Can you work these out from the drawing? Everything is in mm from the part's minimum corner. Give positions to 0.01 mm unless a question says otherwise; leave off trailing zeros. Loops run counter-clockwise (first coordinate to the right, second up) from the corner with the lowest first, then second, coordinate; pieces in that order, holes last. Notation, with made-up numbers: M 33.5,3 L 63.5,3 A10 cw 63.5,10 Z; hole C 36,-10 d4. An arc over 180 degrees is marked long. Use CSV: the item, a comma, the result in double quotes.
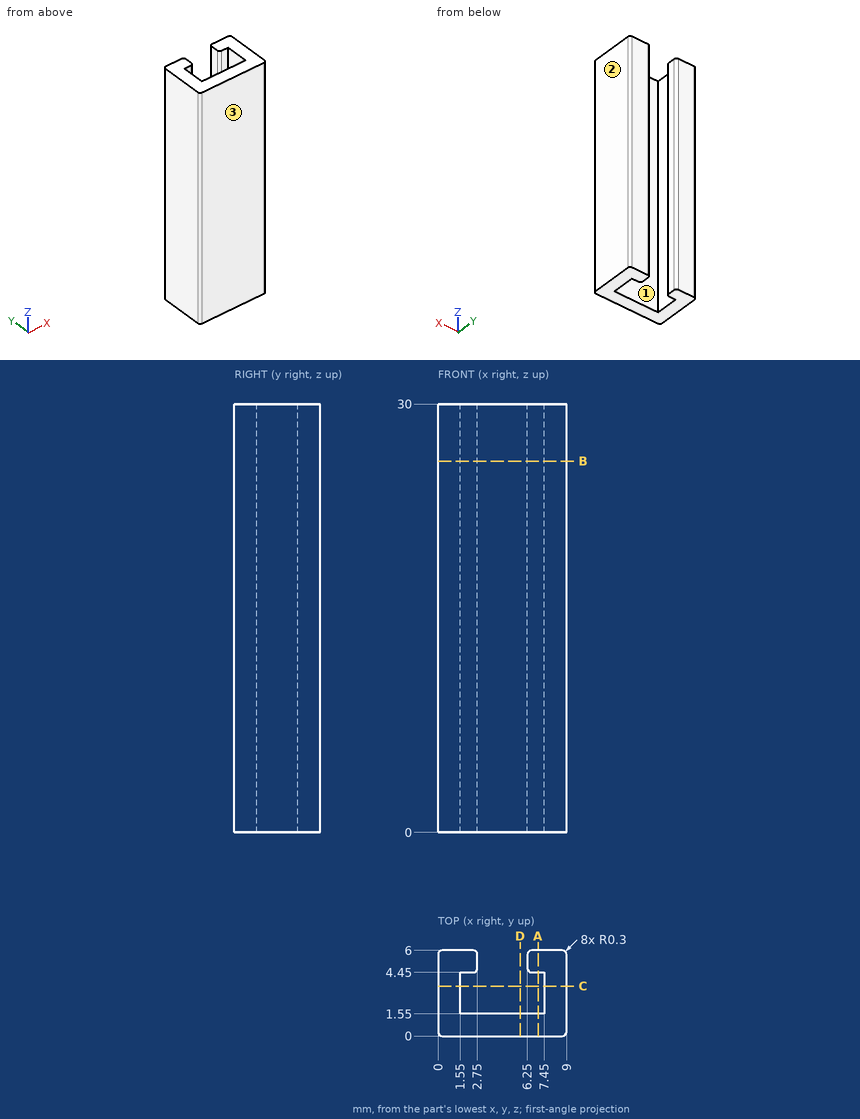
Q1. If we mould it in two halves opening along X, with no side actions, what happens to the marked faces 1, 2 and 3? For each: released by +X, released by -X, zero draft, split by the parting line, or undercut.
Model answer:
face 1,"undercut"
face 2,"released by +X"
face 3,"zero draft"
Q2. I want a section at A-A, the plane x = 7. Please give me the cut outline in (y, z).
Model answer:
outline,"M 0,0 L 1.55,0 L 1.55,30 L 0,30 Z; M 4.45,0 L 6,0 L 6,30 L 4.45,30 Z"
Q3. Please list where these lines run through material, in increasing order: L1, parallel to Y at x = 7, z = 18.5; L2, parallel to X at y = 4.25, z = 18.5; L3, parallel to X at y = 5, z = 7.5. Write a range as from..to.
Model answer:
L1,"0..1.55, 4.45..6"
L2,"0..1.55, 7.45..9"
L3,"0..2.75, 6.25..9"
Q4. I want a section at D-D, the plane x = 5.75. Please give me the cut outline in (y, z), then the cut area to 3 significant figures.
Model answer:
outline,"M 0,0 L 1.55,0 L 1.55,30 L 0,30 Z"
area,"46.5 mm2"
Q5. I want a section at C-C, the plane y = 3.5. Please give me the cut outline in (x, z).
Model answer:
outline,"M 0,0 L 1.55,0 L 1.55,30 L 0,30 Z; M 7.45,0 L 9,0 L 9,30 L 7.45,30 Z"
Q6. I'm going to push a flat-ended pin straight in: P1, Ø1, axis at y = 5.5, z = 21, coming from the -X side. Where does the tip first touch, or does it pass through?
Model answer:
P1,"x = 0"
Q7. I want a section at B-B, the plane z = 26. Please give me the cut outline in (x, y).
Model answer:
outline,"M 0,0.3 A0.3 ccw 0.3,0 L 8.7,0 A0.3 ccw 9,0.3 L 9,5.7 A0.3 ccw 8.7,6 L 6.55,6 A0.3 ccw 6.25,5.7 L 6.25,4.75 A0.3 ccw 6.55,4.45 L 7.45,4.45 L 7.45,1.55 L 1.55,1.55 L 1.55,4.45 L 2.45,4.45 A0.3 ccw 2.75,4.75 L 2.75,5.7 A0.3 ccw 2.45,6 L 0.3,6 A0.3 ccw 0,5.7 Z"
